from build123d import *

# Parameters (mm, degrees)
BOSS_EXTRUDE3_DEPTH = 76.2
SKETCH5_R           = 7.5
CUT_EXTRUDE3_DEPTH  = 149


with BuildPart() as part:
    # Sketch1 → Boss-Extrude3 (new body)
    with BuildSketch(Plane(origin=(0, 0, 0), x_dir=(1, 0, 0), z_dir=(0, 1, 0))):
        with BuildLine():
            Line((-616.834962438, -11.529604763), (-605.550644545, -21.412123117))
            ThreePointArc((-605.550644545, -21.412123117), (-643.422534006, 29.598742869), (-630.001110861, -32.499999959))
            ThreePointArc((-630.001110861, -32.499999959), (0, -148), (630.001110861, -32.499999959))
            ThreePointArc((630.001110861, -32.499999959), (643.422534006, 29.598742869), (605.550644545, -21.412123117))
            Line((605.550644545, -21.412123117), (616.834962438, -11.529604763))
            ThreePointArc((616.834962438, -11.529604763), (637.227790694, 15.937661111), (630, -17.5))
            ThreePointArc((630, -17.5), (0, -133), (-630, -17.5))
            ThreePointArc((-630, -17.5), (-637.227790694, 15.937661111), (-616.834962438, -11.529604763))
        make_face()
    extrude(amount=BOSS_EXTRUDE3_DEPTH)

    # Sketch5 → Cut-Extrude3 (cut, through all)
    with BuildSketch(Plane.XY):
        with Locations((0, 38.1)):
            Circle(SKETCH5_R)
    extrude(amount=CUT_EXTRUDE3_DEPTH, mode=Mode.SUBTRACT)


solid = part.part
Geometry check sheet. Reference: the model listing, model coordinates, mm. Give positions to 0.01 mm unless a question says otherwise; leave off trailing zeros. Loops run counter-clockwise (first coordinate to the right, second up) from the corner with the lowest first, then second, coordinate; pieces in that order, holes last. Notation, with made-up numbers: M 61,-32.5 L 108,-32.5 A24 ccw 108,0.5 Z; hole C 37,53.25 d2. An arc over 180 degrees is marked long. Write each question's results on one line, items separated by ' | '.
1) Gauge pin test, flat ends, axial feed: pin 1 (5 mm diameter, centred on x = 393.5, y = 25.5, fed in from -Z); pin 2 (5 mm diameter, centred on x = -275, y = 16.5, fed in from -Z); pin 3 (6 mm diameter, centred on x = 367, y = 15.5, fed in from -Z). Record the tip position at first contact, or that the pin passes through.
Answers follow:
pin 1: z = 88.29 | pin 2: z = 111.19 | pin 3: z = 94.03
2) Release check for a two-part mould opening along Z. For faces 1 (the face through (636.62, 37.57, -16.2)), 2 (the face through (-637.83, 37.57, -15.65)), 3 (the face through (-3, 76.2, 138)), 4 (the face through (-9.016, 37.567, 147.977)) record: +Z half, -Z half, draft (parallel to the pull), parting line (faces both ways), or undercut.
Answers follow:
face 1: undercut | face 2: undercut | face 3: draft | face 4: +Z half
3) Section check C-C, the plane x = 234. Record the boundary of the cut face in (y, z).
Answers follow:
outline: M 0,117.52 L 76.2,117.52 L 76.2,132.52 L 0,132.52 Z
4) Section check B-B, the plane x = -279. Record the boundary of the cut face in (y, z).
Answers follow:
outline: M 0,110.95 L 76.2,110.95 L 76.2,125.95 L 0,125.95 Z
5) Thickness scan on line 1 (X direction, y = 48, z = 0); line 2 (Y direction, x = 0, z = 141); line 3 (X direction, y = 23, z = 4.5). Record the ranges inside material, lowest first.
Answers follow:
line 1: -662.5 to -647.5, -612.5 to -597.5, 597.5 to 612.5, 647.5 to 662.5 | line 2: 0 to 30.6, 45.6 to 76.2 | line 3: -662.19 to -646.91, -613.09 to -597.81, 597.81 to 613.09, 646.91 to 662.19
6) Section check A-A, the plane z = 81.5. Record the boundary of the cut face in (x, y).
Answers follow:
outline: M -481.43,0 L -424.58,0 L -424.58,76.2 L -481.43,76.2 Z; M 424.58,0 L 481.43,0 L 481.43,76.2 L 424.58,76.2 Z
